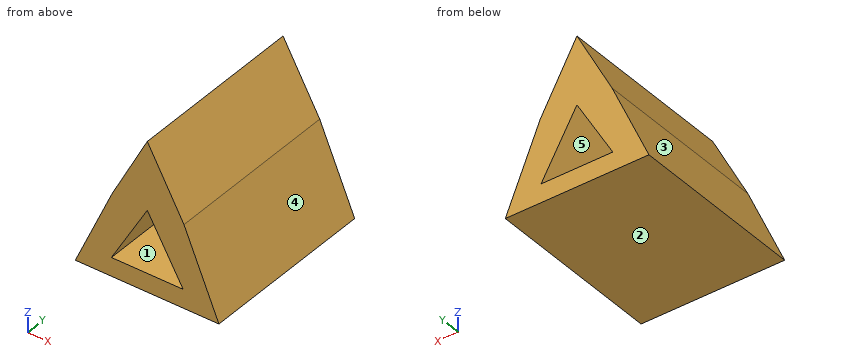
```python
from build123d import *

# Parameters (mm, degrees)
F1_DEPTH = 63.5


with BuildPart() as f1:
    # F0 (on Front) → F1 (new body, symmetric)
    with BuildSketch(Plane.XZ):
        Polygon((-24.8563379985, 28.4985704217), (-50.9303996729, -29.4012854313), (50.6696003271, -29.4012854313), (25.9402706639, 29.0855528694), (0, 75.6930410862), align=None)
        Polygon((0, 27.6665240526), (25.4, -16.3275664596), (-25.4, -16.3275664596), align=None, mode=Mode.SUBTRACT)
    extrude(amount=F1_DEPTH, both=True)


solid = f1.part
```
Geometry check sheet. Reference: the model listing, model coordinates, mm. Face numbers are marked on the shaded views. A direction names the side the tool comes from. Round coordinates to 2 decimals unless told otherwise and drop trailing zeros. Loops run counter-clockwise (first coordinate to the right, second up) from the corner with the lowest first, then second, coordinate; pieces in that order, holes last. Notation, with made-up numbers: (32, 11) - (45, 11) arc R28 cw to (45, 43) - close; hole circle Ø10 at (17, 15). An arc over 180 degrees is marked (long way). Write item = value, one per line. Start each with the question number.
1. Depth check by flat-ended pin: pin 1 (10 mm diameter, centred on y = 32.5, z = 21, fed in from -X); pin 2 (1.5 mm diameter, centred on x = 22.5, y = 4, fed in from +Z); pin 3 (12 mm diameter, centred on y = -8.5, z = 52.5, fed in from -X). Enter the tip coordinate at first touch or a pass-through.
2. Section check A-A on y = -4. Enter the section's corners in (x, z).
3. Section check B-B on z = 14. Enter the section's corners in (x, y).
4. Mould release check, pull along X, two halves, no side actions. Record for the marked faces 3, 4 and 5: released by +X, released by -X, zero draft, split by the parting line, or undercut.
5. Thickness scan on line 1 (X direction, y = 27.5, z = -6.5); line 2 (Z direction, x = -24.5, y = -8); line 3 (Z direction, x = -23, y = -19). Record the ranges inside material, lowest first.
6. Set-up check for the marked faces 1 and 2: record each of +Z, -Z, +X, -X, +Y, -Y from which the full face is reachable in a straight line by a thin tool's end or side.
7. Section check D-D on x = -36. Enter the section's corners in (y, z).
8. Section check C-C on x = 19. Enter the section's corners in (y, z).
Working result:
q1.pin_1 = -30.48
q1.pin_2 = 36.61
q1.pin_3 = -15.38
q2.outline = (-50.93, -29.4) - (50.67, -29.4) - (25.94, 29.09) - (0, 75.69) - (-24.86, 28.5) - close; hole (-25.4, -16.33) - (25.4, -16.33) - (0, 27.67) - close
q3.outline = (-31.39, -63.5) - (-7.89, -63.5) - (-7.89, 63.5) - (-31.39, 63.5) - close; (7.89, -63.5) - (32.32, -63.5) - (32.32, 63.5) - (7.89, 63.5) - close
q4.face_3 = released by -X
q4.face_4 = released by +X
q4.face_5 = undercut
q5.line_1 = -40.62 to -19.73, 19.73 to 40.99
q5.line_2 = -29.4 to -16.33, -14.77 to 29.18
q5.line_3 = -29.4 to -16.33, -12.17 to 32.02
q6.face_1 = +Y, -Y
q6.face_2 = -Z, +X, -X, +Y, -Y
q7.outline = (-63.5, -29.4) - (63.5, -29.4) - (63.5, 3.75) - (-63.5, 3.75) - close
q8.outline = (-63.5, -29.4) - (63.5, -29.4) - (63.5, -16.33) - (-63.5, -16.33) - close; (-63.5, -5.24) - (63.5, -5.24) - (63.5, 41.56) - (-63.5, 41.56) - close
